Verification items for this drawing (mm, ordinates from the low corner). A direction names the side the tool comes from. Round coordinates to 2 decimals unless told otherwise and drop trailing zeros. Order: outer loops, then holes, each group sorted by start corner. A loop starts at its lowest first (then second) coordinate and runs counter-clockwise, first axis right, second up. Notation, with made-up numbers: (-2.75, 18.25) -> (6.25, 18.25) arc R34 cw to (6.25, 51.25) -> close; hole circle Ø8 at (-1, 51). An arc over 180 degrees is marked (long way). Answer in a Markdown table with one row per item.
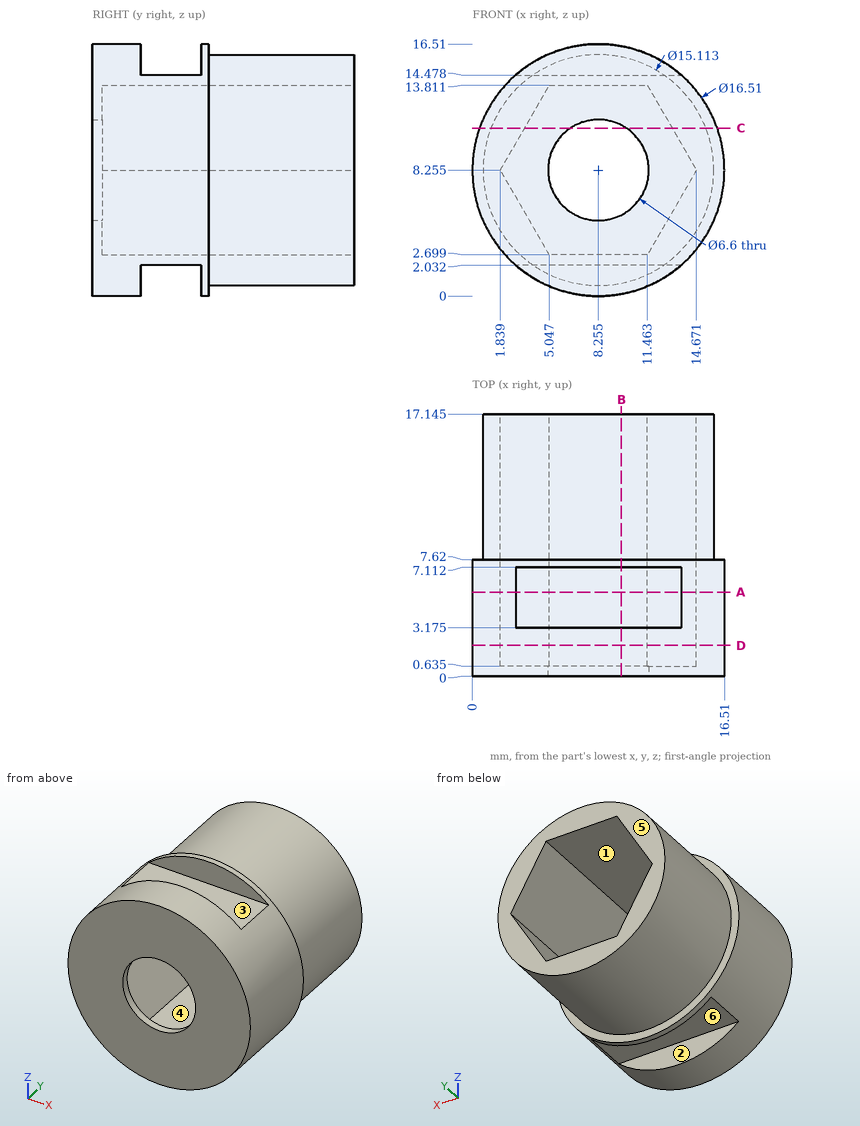
Item 1: Cross-section at B-B (x = 9.75). Record the boundary of the cut face in (y, z) (1 decimal).
Result sheet:
| item | result |
|---|---|
| outline | (0, 0.1) -> (3.2, 0.1) -> (3.2, 2) -> (7.1, 2) -> (7.1, 0.1) -> (7.6, 0.1) -> (7.6, 0.8) -> (17.1, 0.8) -> (17.1, 2.7) -> (0.6, 2.7) -> (0.6, 5.3) -> (0, 5.3) -> close; (0, 11.2) -> (0.6, 11.2) -> (0.6, 13.8) -> (17.1, 13.8) -> (17.1, 15.7) -> (7.6, 15.7) -> (7.6, 16.4) -> (7.1, 16.4) -> (7.1, 14.5) -> (3.2, 14.5) -> (3.2, 16.4) -> (0, 16.4) -> close |
Item 2: Cross-section at A-A (y = 5.5). Record the boundary of the cut face in (x, z) (1 decimal).
Result sheet:
| item | result |
|---|---|
| outline | (2.8, 2) -> (13.7, 2) arc R8.3 ccw to (13.7, 14.5) -> (2.8, 14.5) arc R8.3 ccw to start; hole (1.8, 8.3) -> (5, 2.7) -> (11.5, 2.7) -> (14.7, 8.3) -> (11.5, 13.8) -> (5, 13.8) -> close |
Item 3: Mould release check, pull along Y, two halves, no side actions. Record for the marked faces 4, 5 and 6: pulls with the +Y half, pulls with the -Y half, needs draft (parallel to the pull), parting line crosses it, or undercut.
Result sheet:
| item | result |
|---|---|
| face 4 | needs draft |
| face 5 | pulls with the +Y half |
| face 6 | undercut |
Item 4: Depth check by flat-ended pin: P1, Ø2, axis at y = 11.5, z = 9.5, coming from the -X side; P2, Ø2, axis at x = 5.5, y = 4, coming from the -Z side; P3, Ø2, axis at x = 7, y = 4.5, coming from the +Z side; P4, Ø4, axis at x = 8.255, z = 8.255, coming from the -Y side. Enter the tip coordinate at first touch or a pass-through.
Result sheet:
| item | result |
|---|---|
| P1 | stops at x = 0.7 |
| P2 | stops at z = 0.3 |
| P3 | stops at z = 14.48 |
| P4 | passes through |
Item 5: Set-up check for the marked faces 1, 2 and 3: record each of +Z, -Z, +X, -X, +Y, -Y from which the full face is reachable in a straight line by a thin tool's end or side.
Result sheet:
| item | result |
|---|---|
| face 1 | +Y |
| face 2 | -Z, +X, -X |
| face 3 | +Z, +X, -X |
Item 6: Cross-section at C-C (z = 11). Record the boundary of the cut face in (x, y) (1 decimal).
Result sheet:
| item | result |
|---|---|
| outline | (0.5, 0) -> (6.4, 0) -> (6.4, 0.6) -> (3.4, 0.6) -> (3.4, 17.1) -> (1.2, 17.1) -> (1.2, 7.6) -> (0.5, 7.6) -> close; (10.1, 0) -> (16, 0) -> (16, 7.6) -> (15.3, 7.6) -> (15.3, 17.1) -> (13.1, 17.1) -> (13.1, 0.6) -> (10.1, 0.6) -> close |
Item 7: Cross-section at D-D (y = 2). Record the boundary of the cut face in (x, z) (1 decimal), and give its area (3 significant figures).
Result sheet:
| item | result |
|---|---|
| outline | circle Ø16.5 at (8.3, 8.3); hole (1.8, 8.3) -> (5, 2.7) -> (11.5, 2.7) -> (14.7, 8.3) -> (11.5, 13.8) -> (5, 13.8) -> close |
| area | 107 mm^2 |
Item 8: Scan lines: line 1 (Z direction, x = 11.25, y = 3.25); line 2 (X direction, y = 15, z = 3.75); line 3 (Z direction, x = 6.5, y = 10) (1 decimal). Record each from-to range of solid material in increasing order. Write a range as [from, to].
Result sheet:
| item | result |
|---|---|
| line 1 | z = [2.03, 2.7], [13.81, 14.48] |
| line 2 | x = [2.19, 4.44], [12.07, 14.32] |
| line 3 | z = [0.9, 2.7], [13.8, 15.6] |
